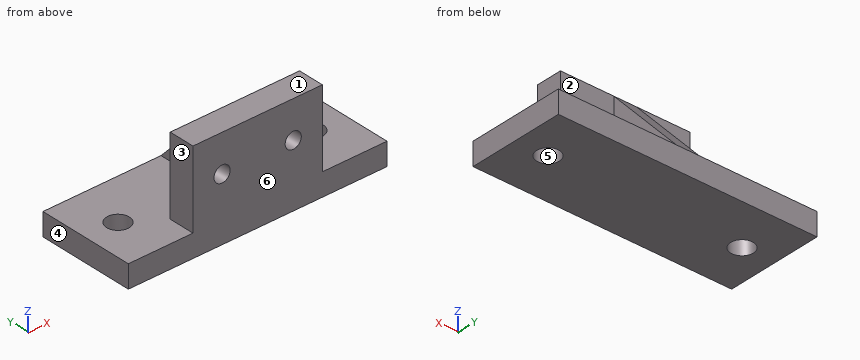
Autodesk Fusion 360 part; units mm, degrees
sketch "Skizze1" plane through (0, 0, 0) normal (0, 0, 1) x (1, 0, 0)
  line L0 (0, 0) -> (80, 0)
  line L1 (80, 0) -> (80, 30)
  line L2 (80, 30) -> (0, 30)
  line L3 (0, 30) -> (0, 0)
  line L4 (0, 30) -> (10, 30)
  line L5 (10, 30) -> (10, 15)
  line L6 (10, 15) -> (0, 15)
  line L7 (0, 15) -> (0, 30)
  line L8 (80, 30) -> (70, 30)
  line L9 (70, 30) -> (70, 15)
  line L10 (70, 15) -> (80, 15)
  line L11 (80, 15) -> (80, 30)
  circle A0 centre (10, 15) radius 3.5
  circle A1 centre (70, 15) radius 3.5
  dimension "d1" = 80
  dimension "d2" = 30
  dimension "d3" = 10
  dimension "d4" = 15
  dimension "d5" = 10
  dimension "d6" = 15
  dimension "d7" = 7
  dimension "d8" = 7
extrude "Extrusion1" add sketch "Skizze1" along normal blind 7 contours L0 L1 L2 L3 L5 L6 L9 L10 A0 A1 | L2 L3 L4 L5 L6 L7 A0 | L1 L2 L8 L9 L10 L11 A1
sketch "Skizze2" plane through (0, 0, 0) normal (0, 1, 0) x (1, 0, 0)
sketch "Skizze3" plane through (0, 0, 7) normal (0, 0, 1) x (-1, 0, 0)
  circle A0 centre (-70, -15) radius 3.5
  circle A1 centre (-10, -15) radius 3.5
  line L0 (0, -30) -> (0, 0)
  line L1 (0, 0) -> (-80, 0)
  line L2 (-80, 0) -> (-80, -30)
  line L3 (-80, -30) -> (0, -30)
  line L4 (0, 0) -> (-80, 0)
  line L5 (-80, 0) -> (-80, -5)
  line L6 (-80, -5) -> (0, -5)
  line L7 (0, -5) -> (0, 0)
  dimension "d11" = 5
extrude "Extrusion2" add sketch "Skizze3" along normal blind 24 contours L0 L1 L2 L4 L5 L6 L7
sketch "Skizze4" plane through (0, 0, 0) normal (0, -1, 0) x (1, 0, 0)
  line L0 (0, 0) -> (80, 0)
  line L1 (80, 0) -> (80, 31)
  line L2 (80, 31) -> (0, 31)
  line L3 (0, 31) -> (0, 0)
  line L4 (40, 31) -> (40, 19)
  line L5 (40, 0) -> (40, 19.5)
  line L6 (40, 19.5) -> (51, 19.5)
  circle A0 centre (51, 19.5) radius 2.5
  line L7 (40, 19.5) -> (29, 19.5)
  circle A1 centre (29, 19.5) radius 2.5
  dimension "d37" = 19.5
  dimension "d38" = 11
  dimension "d39" = 5
  dimension "d40" = 11
  dimension "d41" = 5
extrude "Extrusion10" cut sketch "Skizze4" against normal blind 9 contours A1 | A0
extrude "Extrusion11" add 1 faces at (8.8333, 5, 19.1667) along direction (0, 1, 0) blind 3
sketch "Skizze8" plane through (80, 0, 0) normal (1, 0, 0) x (0, 1, 0)
  line L0 (0, 0) -> (30, 0)
  line L1 (30, 0) -> (30, 7)
  line L2 (30, 7) -> (8, 7)
  line L3 (8, 7) -> (8, 31)
  line L4 (8, 31) -> (0, 31)
  line L5 (0, 31) -> (0, 0)
  line L6 (0, 31) -> (8, 31)
  line L7 (8, 31) -> (8, 7)
  line L8 (8, 7) -> (0, 7)
  line L9 (0, 7) -> (0, 31)
extrude "Extrusion12" cut sketch "Skizze8" against normal blind 20 contours L3 L4 L5 L6 L7 L8 L9
sketch "Skizze9" plane through (0, 0, 0) normal (-1, 0, 0) x (0, -1, 0)
  line L0 (-30, 0) -> (0, 0)
  line L1 (0, 0) -> (0, 31)
  line L2 (0, 31) -> (-8, 31)
  line L3 (-8, 31) -> (-8, 7)
  line L4 (-8, 7) -> (-30, 7)
  line L5 (-30, 7) -> (-30, 0)
  line L6 (0, 31) -> (-8, 31)
  line L7 (-8, 31) -> (-8, 7)
  line L8 (-8, 7) -> (0, 7)
  line L9 (0, 7) -> (0, 31)
extrude "Extrusion13" cut sketch "Skizze9" against normal blind 20 contours L1 L2 L3 L6 L7 L8 L9
sketch "Skizze10" plane through (0, 0, 7) normal (0, 0, 1) x (-1, 0, 0)
  circle A0 centre (-10, -15) radius 3.5
  circle A1 centre (-70, -15) radius 3.5
  line L0 (-20, -8) -> (-60, -8)
  line L1 (-60, -8) -> (-60, 0)
  line L2 (-60, 0) -> (-80, 0)
  line L3 (-80, 0) -> (-80, -30)
  line L4 (-80, -30) -> (0, -30)
  line L5 (0, -30) -> (0, 0)
  line L6 (0, 0) -> (-20, 0)
  line L7 (-20, 0) -> (-20, -8)
  line L8 (-40, -30) -> (-36.5, -30)
  line L9 (-36.5, -30) -> (-43.5, -30)
  line L10 (-43.5, -30) -> (-43.5, -8)
  line L11 (-43.5, -8) -> (-36.5, -8)
  line L12 (-36.5, -8) -> (-36.5, -30)
  dimension "d52" = 3.5
  dimension "d53" = 7
extrude "Extrusion14" add sketch "Skizze10" along normal blind 24 contours L0 L4 L8 L9 L10 L11 L12
chamfer "Fase3" distance 22 distance2 24 1 edges at (40, 30, 31) measured on face at (41.1667, 2.6667, 31)
The listing builds one solid part. Answer for the finished solid, in the listing's coordinates (mm). Face numbers are marked on the shaded views. A direction names the side the tool comes from. Round coordinates to 2 decimals unless told otherwise and drop trailing zeros. Loops run counter-clockwise (first coordinate to the right, second up) from the corner with the lowest first, then second, coordinate; pieces in that order, holes last. Notation, with made-up numbers: M -39.5,-37.75 L -18.5,-37.75 A36 ccw -18.5,-1.75 Z; hole C -10,64 d11. An arc over 180 degrees is marked long. Return JSON: item names as keys, results as strings.
Q1. Each of these flat-tipped pins is pushed along its axis until it touches: pin 1 Ø11 at (y, z) = (17.5, 18.5) entering from -X; pin 2 Ø1.5 at (x, z) = (26, 21) entering from +Y; pin 3 Ø2.5 at (y, z) = (3.5, 19) entering from +X; pin 4 Ø3 at (x, z) = (29, 19.5) entering from -Y. Where does it stop, or does it pass through?
Results list:
{"pin 1": "stops at x = 36.5", "pin 2": "stops at y = 8", "pin 3": "stops at x = 60", "pin 4": "passes through"}
Q2. Find section B-B, the plane y = 5.5. Determine the outline of the cut face in (x, z), plus the area to 3 significant figures.
Results list:
{"outline": "M 0,0 L 80,0 L 80,7 L 60,7 L 60,31 L 20,31 L 20,7 L 0,7 Z; hole C 29,19.5 d5; hole C 51,19.5 d5", "area": "1,480 mm2"}
Q3. Find section C-C, the plane z = 25. Determine the outline of the cut face in (x, y), plus the area to 4 significant figures.
Results list:
{"outline": "M 20,0 L 60,0 L 60,8 L 43.5,8 L 43.5,13.5 L 36.5,13.5 L 36.5,8 L 20,8 Z", "area": "358.5 mm2"}
Q4. The mould has two halves that part along X. Classify the marked faces 4, 5 and 6: released by +X, released by -X, zero draft, split by the parting line, or undercut.
Results list:
{"face 4": "released by -X", "face 5": "undercut", "face 6": "zero draft"}
Q5. Which of the six approach directions +Z, -Z, +X, -X, +Y, -Y give full straight-line access (tool end or side, diameter ignored) to the marked faces 1, 2 and 3?
Results list:
{"face 1": "+Z, +X, -X, +Y, -Y", "face 2": "+Z, +X, +Y", "face 3": "+Z, -X, +Y, -Y"}
Q6. Find section D-D, the plane z = 19.5. Determine the outline of the cut face in (x, y).
Results list:
{"outline": "M 20,0 L 26.5,0 L 26.5,8 L 20,8 Z; M 31.5,0 L 48.5,0 L 48.5,8 L 43.5,8 L 43.5,18.54 L 36.5,18.54 L 36.5,8 L 31.5,8 Z; M 53.5,0 L 60,0 L 60,8 L 53.5,8 Z"}
Q7. Find the intervals of material crossed by line 1 along X through (y, z) = (15, 2); line 2 along Z through (x, y) = (51, 3.5); line 3 along Y through (x, z) = (10, 5), in increasing order. Write a range as from..to.
Results list:
{"line 1": "x = 0..6.5, 13.5..66.5, 73.5..80", "line 2": "z = 0..17, 22..31", "line 3": "y = 0..11.5, 18.5..30"}
Q8. Find section A-A, the plane x = 70. Determine the outline of the cut face in (y, z), plus the area to 3 significant figures.
Results list:
{"outline": "M 0,0 L 11.5,0 L 11.5,7 L 0,7 Z; M 18.5,0 L 30,0 L 30,7 L 18.5,7 Z", "area": "161 mm2"}
